For this review, take the finished solid that the model builds, in its own axes (mm). Face numbers are marked on the shaded views. A direction names the side the tool comes from. Round coordinates to 2 decimals unless told otherwise and drop trailing zeros. Order: outer loops, then holes, each group sorted by start corner. A loop starts at its lowest first (then second) coordinate and runs counter-clockwise, first axis right, second up.
Autodesk Inventor part; units mm, degrees
ref_plane "YZ Plane" through (0, 0, 0) normal (1, 0, 0) x (0, 1, 0)
ref_plane "XZ Plane" through (0, 0, 0) normal (0, 1, 0) x (-1, 0, 0)
ref_plane "XY Plane" through (0, 0, 0) normal (0, 0, 1) x (1, 0, 0)
sketch "Sketch1" plane through (0, 0, 0) normal (0, 0, 1) x (1, 0, 0)
  line L0 (-20, -7.5) -> (20, -7.5)
  line L1 (20, -7.5) -> (20, 7.5)
  line L2 (20, 7.5) -> (-20, 7.5)
  line L3 (-20, 7.5) -> (-20, -7.5)
  line L4 (-20, -7.5) -> (20, 7.5) construction
  line L5 (20, -7.5) -> (-20, 7.5) construction
  point P0 (0, 0)
  dimension "d0" = 15
  dimension "d1" = 40
extrude "Extrusion1" add sketch "Sketch1" along normal blind 10.75
sketch "Sketch2" plane through (0, 0, 10.75) normal (0, 0, 1) x (1, 0, 0)
  line L0 (-20, 7.5) -> (-20, -7.5) construction
  line L1 (-20, 0) -> (-13, 0) construction
  line L2 (-13, 0) -> (-3, 0) construction
  circle A0 centre (-13, 0) radius 2.25
  circle A1 centre (-3, 0) radius 2.25
  point P0 (0, 0)
  dimension "d4" = 10
  dimension "d5" = 7
  dimension "d6" = 4.5
extrude "Extrusion2" cut sketch "Sketch2" against normal through all
sketch "Sketch3" plane through (0, 0, 10.75) normal (0, 0, 1) x (1, 0, 0)
  circle A0 centre (-13, 0) radius 2.25
  circle A1 centre (-13, 0) radius 4
  circle A2 centre (-3, 0) radius 2.25
  circle A3 centre (-3, 0) radius 4
  point P0 (0, 0)
  dimension "d9" = 8
extrude "Extrusion3" cut sketch "Sketch3" against normal blind 5 contours A0 | A1 | A2 | A3
sketch "Sketch4" plane through (0, 0, 0) normal (0, 0, -1) x (-1, 0, 0)
  line L0 (-20, -7.5) -> (-20, 7.5) construction
  line L1 (-20, 0) -> (-13, 0) construction
  circle A0 centre (-13, 0) radius 2.75
  point P0 (0, 0)
  dimension "d12" = 5.5
  dimension "d13" = 7
extrude "Extrusion4" cut sketch "Sketch4" against normal through all
sketch "Sketch5" plane through (0, 0, 0) normal (0, 0, -1) x (-1, 0, 0)
  circle A0 centre (-13, 0) radius 2.75
  circle A1 centre (-13, 0) radius 4.75
  point P0 (0, 0)
  dimension "d16" = 9.5
extrude "Extrusion5" cut sketch "Sketch5" against normal blind 6 contours A0 | A1
sketch "Sketch6" plane through (13, 0, 6) normal (0, 0, -1) x (-1, 0, 0)
  line L0 (5.3295, 6.8206) -> (-5.8691, 6.8206)
  line L1 (-5.8691, 6.8206) -> (-5.8691, 2.75)
  line L2 (-5.8691, 2.75) -> (5.3295, 2.75)
  line L3 (5.3295, 2.75) -> (5.3295, 6.8206)
  line L4 (6.0982, -2.75) -> (-4.6287, -2.75)
  line L5 (-4.6287, -2.75) -> (-4.6287, -7.6942)
  line L6 (-4.6287, -7.6942) -> (6.0982, -7.6942)
  line L7 (6.0982, -7.6942) -> (6.0982, -2.75)
  circle A0 centre (0, 0) radius 2.75
  circle A1 centre (0, 0) radius 4.75
  point P0 (13, 0)
  point P1 (-3.873, 2.75)
  point P2 (-3.873, -2.75)
  point P3 (0, -2.75)
  point P4 (0, 2.75)
  point P5 (3.873, 2.75)
  point P6 (3.873, -2.75)
extrude "Extrusion6" cut sketch "Sketch6" against normal blind 0.2 contours A1 L4 A0 L2 | L2 A0 L4 A1
sketch "Sketch7" plane through (13, 0, 6.2) normal (0, 0, -1) x (-1, 0, 0)
  line L0 (3.873, -2.75) -> (0, -2.75)
  arc A0 (3.873, -2.75) -> (3.873, 2.75) centre (0, 0) ccw
  line L1 (0, 2.75) -> (3.873, 2.75)
  arc A1 (0, -2.75) -> (0, 2.75) centre (0, 0) ccw
  line L2 (-3.873, 2.75) -> (0, 2.75)
  arc A2 (-3.873, 2.75) -> (-3.873, -2.75) centre (0, 0) ccw
  line L3 (0, -2.75) -> (-3.873, -2.75)
  arc A3 (0, 2.75) -> (0, -2.75) centre (0, 0) ccw
  line L4 (7.5317, 4.6908) -> (2.75, 4.6908)
  line L5 (2.75, 4.6908) -> (2.75, -4.4637)
  line L6 (2.75, -4.4637) -> (7.5317, -4.4637)
  line L7 (7.5317, -4.4637) -> (7.5317, 4.6908)
  line L8 (-5.9646, 6.0361) -> (-2.75, 6.0361)
  line L9 (-2.75, 6.0361) -> (-2.75, -5.4071)
  line L10 (-2.75, -5.4071) -> (-5.9646, -5.4071)
  line L11 (-5.9646, -5.4071) -> (-5.9646, 6.0361)
  arc A4 (0, -2.75) -> (0, 2.75) centre (0, 0) ccw
  point P0 (13, 0)
  point P1 (-2.75, 2.75)
  point P2 (-2.75, 0)
  point P3 (2.75, 0)
  point P4 (2.75, 2.75)
  point P5 (2.75, -2.75)
  point P6 (-2.75, -2.75)
extrude "Extrusion7" cut sketch "Sketch7" against normal blind 0.2 contours L0 A1 L5 | L3 L9 A3 | A1 L1 L5 | L9 L2 A3
properties part number "LoadCellMount"
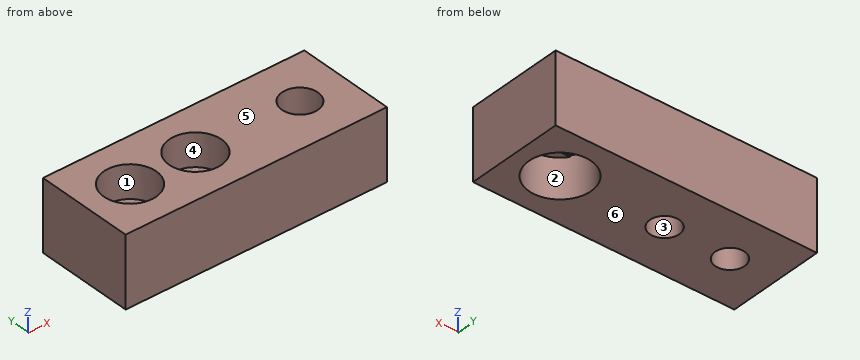
(1) Add section D-D on z = 1.5. Give the boundary of the cut face in (x, y).
(2) Add section A-A on z = 9. Give the boundary of the cut face in (x, y), plus the area to 3 significant figures.
(3) Draft analysis for pull direction Z (two halves, no side actions). For the marked faces 4, 5 and 6, state which applies: pulls with the +Z half, pulls with the -Z half, needs draft (parallel to the pull), parting line crosses it, or undercut.
(4) Wall thickness on L1, parallel to Y at x = -13, z = 9.2; L2, parallel to Y at x = -13, z = 3.3; L3, parallel to X at y = 2.5, z = 10.5: over which ranges is each line inside the solid? List them lowest first.
(5) Tool access review of the marked faces 1, 2 and 3: name each direction out of +Z, -Z, +X, -X, +Y, -Y from which nothing blocks a thin tool from reaching the whole face with its end or side.
(6) Add section B-B on x = -3. Give the boundary of the cut face in (y, z).
(7) Clearance check with flat-ended pins moving along their axes: P1, Ø1.4, axis at x = 14.5, y = 1.5, coming from the -Z side; P2, Ø3, axis at x = 11.5, y = 1.5, coming from the -Z side; P3, Ø6.5, axis at x = -3.5, y = 0, coming from the +Z side; P4, Ø3.5, axis at x = -13, y = 0, coming from the +Z side (3 decimals). State where each tip first meets the part, or that it passes through.
(8) Add section C-C on y = 0.5. Count the separate pieces of the cut face and the enclosed holes in it, plus the area to 3 significant figures.
Here are the results:
1. outline: (-20, -7.5) - (20, -7.5) - (20, 7.5) - (-20, 7.5) - close; hole circle Ø4.5 at (-13, 0); hole circle Ø4.5 at (-3, 0); hole circle Ø9.5 at (13, 0)
2. outline: (-20, -7.5) - (20, -7.5) - (20, 7.5) - (-20, 7.5) - close; hole circle Ø8 at (-13, 0); hole circle Ø8 at (-3, 0); hole circle Ø5.5 at (13, 0)
2. area: 476 mm2
3. face 4: needs draft
3. face 5: pulls with the +Z half
3. face 6: pulls with the -Z half
4. L1: y = -7.5 to -4, 4 to 7.5
4. L2: y = -7.5 to -2.25, 2.25 to 7.5
4. L3: x = -20 to -16.12, -9.88 to -6.12, 0.12 to 11.85, 14.15 to 20
5. face 1: +Z
5. face 2: -Z
5. face 3: +Z, -Z
6. outline: (-7.5, 0) - (-2.25, 0) - (-2.25, 5.75) - (-4, 5.75) - (-4, 10.75) - (-7.5, 10.75) - close; (2.25, 0) - (7.5, 0) - (7.5, 10.75) - (4, 10.75) - (4, 5.75) - (2.25, 5.75) - close
7. P1: stops at z = 6.4
7. P2: stops at z = 6
7. P3: stops at z = 5.75
7. P4: passes through
8. separate pieces: 4
8. enclosed holes: 0
8. area: 217 mm2
